Autodesk Inventor part; units mm, degrees
ref_plane "YZ Plane" through (0, 0, 0) normal (1, 0, 0) x (0, 1, 0)
ref_plane "XZ Plane" through (0, 0, 0) normal (0, 1, 0) x (-1, 0, 0)
ref_plane "XY Plane" through (0, 0, 0) normal (0, 0, 1) x (1, 0, 0)
sketch "Sketch1" plane through (0, 0, 0) normal (0, 0, 1) x (1, 0, 0)
  line L0 (0, 0) -> (24, 0)
  line L1 (24, 0) -> (24, -100)
  line L2 (24, -100) -> (0, -100)
  line L3 (0, -100) -> (0, 0)
  dimension "d0" = 24
  dimension "d1" = 100
extrude "Extrusion1" add sketch "Sketch1" along normal blind 2
sketch "Sketch2" plane through (0, 0, 2) normal (0, 0, 1) x (1, 0, 0)
  line L0 (0, -100) -> (24, -100)
  line L1 (0, 0) -> (2, 0)
  line L2 (2, 0) -> (2, -100)
  line L3 (2, -100) -> (0, -100)
  line L4 (0, -100) -> (0, 0)
  line L5 (24, -100) -> (24, 0)
  line L6 (24, 0) -> (22, 0)
  line L7 (22, 0) -> (22, -100)
  line L8 (22, -100) -> (24, -100)
  line L9 (24, -100) -> (24, 0)
  dimension "d4" = 2
  dimension "d5" = 2
extrude "Extrusion2" add sketch "Sketch2" along normal blind 15
sketch "Sketch3" plane through (24, -100, 0) normal (1, 0, 0) x (0, 0, -1)
  circle A0 centre (-8.5, 97) radius 1
  circle A1 centre (-8.5, 69.5) radius 1
  line L0 (-17, 0) -> (-17, 100)
  line L1 (0, 100) -> (-17, 100)
  dimension "d8" = 2
  dimension "d9" = 2
  dimension "d10" = 8.5
  dimension "d11" = 8.5
  dimension "d12" = 27.5
  dimension "d13" = 3
extrude "Extrusion3" cut sketch "Sketch3" against normal up to surface (2 mm away)
sketch "Sketch4" plane through (24, -100, 0) normal (1, 0, 0) x (0, 0, -1)
  line L0 (-17, 100) -> (-17, 0)
  line L1 (-2, 95) -> (-2, 71.5)
  circle A0 centre (-8.5, 97) radius 1
  circle A1 centre (-8.5, 69.5) radius 1
  line L2 (0, 0) -> (0, 100)
  line L3 (-2, 95) -> (-17, 95)
  line L4 (-17, 95) -> (-17, 71.5)
  line L5 (-17, 71.5) -> (-2, 71.5)
  point P0 (-17, 95)
  dimension "d24" = 23.5
  dimension "d104" = 15
  dimension "d105" = 2
  dimension "d106" = 2
extrude "Extrusion4" cut sketch "Sketch4" against normal up to surface (2 mm away) contours L3 L1 L5 L0
sketch "Sketch5" plane through (0, -100, 0) normal (-1, 0, 0) x (0, 0, 1)
  circle A0 centre (8.5, 88.4) radius 2.5
  circle A1 centre (8.5, 97) radius 1
  point P0 (0, 100)
  dimension "d29" = 5
  dimension "d32" = 8.6
  dimension "d33" = 0
extrude "Extrusion5" add sketch "Sketch5" along normal blind 5 contours A0
sketch "Sketch15" plane through (0, 0, 0) normal (0, 1, 0) x (1, 0, 0)
  line L0 (22, -17) -> (24, -17)
  line L1 (0, 0) -> (0, -17)
  line L2 (24, -17) -> (0, -17)
  line L3 (0, -17) -> (0, 0)
  line L4 (0, 0) -> (24, 0)
  line L5 (24, 0) -> (24, -17)
extrude "Extrusion12" add sketch "Sketch15" along normal blind 2
sketch "Sketch16" plane through (24, -100, 17) normal (1, 0, 0) x (0, 0, -1)
  line L0 (0, 100) -> (0, 0)
  line L1 (0, 5) -> (15, 5)
  line L2 (15, 5) -> (15, 28.5)
  line L3 (15, 28.5) -> (0, 28.5)
  line L4 (0, 28.5) -> (0, 5)
  line L5 (17, 0) -> (0, 0)
  circle A0 centre (8.5, 3) radius 1
  circle A1 centre (8.5, 30.5) radius 1
  point P0 (17, 100)
  point P1 (0, 71.5)
  point P2 (7.5, 5)
  point P3 (7.5, 28.5)
  point P4 (0, 28.5)
  dimension "d84" = 15
  dimension "d85" = 23.5
  dimension "d86" = 5
  dimension "d87" = 2
  dimension "d88" = 2
  dimension "d89" = 8.5
  dimension "d90" = 8.5
  dimension "d91" = 2
  dimension "d92" = 2
extrude "Extrusion13" cut sketch "Sketch16" against normal up to surface (2 mm away)
sketch "Sketch17" plane through (0, -100, 0) normal (0, -1, 0) x (1, 0, 0)
  line L0 (24, 4) -> (24, 17)
  line L1 (24, 17) -> (0, 17)
  line L2 (0, 17) -> (0, 0)
  line L3 (0, 0) -> (24, 0)
  line L4 (24, 0) -> (24, 17)
  point P0 (24, 2)
extrude "Extrusion14" add sketch "Sketch17" along normal blind 2
sketch "Sketch18" plane through (0, 2, 0) normal (-1, 0, 0) x (0, 0, 1)
  circle A0 centre (8.5, -90.4) radius 2.5
  line L0 (17, -104) -> (0, -104)
  line L1 (17, -104) -> (17, 0)
  point P0 (0, -2)
  dimension "d97" = 5
  dimension "d98" = 13.6
  dimension "d99" = 8.5
extrude "Extrusion15" add sketch "Sketch18" along normal blind 5
ref_plane "Plano de trabalho3" through (2, -44.5, 2) normal (1, 0, 0) x (0, 0, -1)
sketch "Sketch21" plane through (2, -44.5, 2) normal (1, 0, 0) x (0, 0, -1)
  circle A0 centre (-6.5, -5.5) radius 6
  line L0 (0, 9) -> (-15, 9)
  line L1 (-15, -35.5) -> (-15, 44.5)
  circle A1 centre (-6.4973, 4.5) radius 1.5
  circle A2 centre (-6.5, -15.5) radius 1.5
  line L2 (0, 44.5) -> (-15, 44.5)
  point P0 (2, 44.5)
  point P1 (-15, 0)
  point P2 (-15, 46.5)
  dimension "d122" = 12
  dimension "d124" = 8.5
  dimension "d129" = 3
  dimension "d130" = 3
  dimension "d131" = 10
  dimension "d132" = 10
  dimension "d134" = 50
extrude "Extrusion18" cut sketch "Sketch21" against normal up to surface (2 mm away)
sketch "Esboço22" plane through (0, 0, 2) normal (0, 0, 1) x (1, 0, 0)
  line L0 (22, -71.5) -> (22, -28.5)
  line L1 (22, -38.5) -> (15, -38.5)
  line L2 (15, -38.5) -> (15, -61.5)
  line L3 (15, -61.5) -> (22, -61.5)
  line L4 (22, -61.5) -> (22, -38.5)
  line L5 (24, -28.5) -> (22, -28.5)
  line L6 (22, -71.5) -> (24, -71.5)
  point P0 (0, 0)
  dimension "d142" = 7
  dimension "d143" = 10
  dimension "d144" = 10
extrude "Extrusão19" add sketch "Esboço22" along normal up to surface (15 mm away)
equation "\"d11\" = d10"
equation "\"d90\" = d89"
properties part number "corpo"
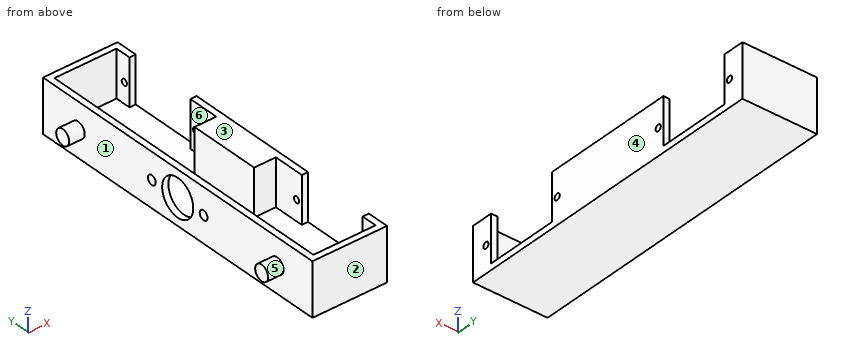
The listing builds one solid part. Answer for the finished solid, in the listing's coordinates (mm). Face numbers are marked on the shaded views. A direction names the side the tool comes from. Coordinates: 2 decimals unless noted, no trailing zeros. Write each loop counter-clockwise with the first axis right and the second up, starting at its lowest first coordinate (ties: lowest second). Pieces come first, ordered by that corner, then holes. Notation, with made-up numbers: M 29.25,8.25 L 55.25,8.25 A37 ccw 55.25,45.25 Z; hole C 0.5,-27.75 d3. An arc over 180 degrees is marked long. Write each question's results on one line, items separated by ' | '.
Item 1: Consider probe 1 along Y at (x, z) = (15.25, 13.5); probe 2 along Y at (x, z) = (10, 13.5); probe 3 along X at (y, z) = (-31, 4.25). Determine where each line is inside the solid, lowest interval first. Write a range as [from, to].
Answer below:
probe 1: [-102, -100], [-61.5, -38.5], [0, 2] | probe 2: [-102, -100], [0, 2] | probe 3: [0, 2], [22, 24]
Item 2: Given P1, Ø1.5, axis at x = 0.5, y = -11, coming from the -Z side; P2, Ø8, axis at y = -23.5, z = 12.5, coming from the +X side; P3, Ø7.5, axis at y = -52.5, z = 6, coming from the -X side, each flat-ended and moving along its own axis, determine where each tip first touches the part or whether it passes through.
Answer below:
P1: z = 0 | P2: x = 2 | P3: x = 0
Item 3: The part is cut by section D-D on y = -50. Determine the outline of the cut face in (x, z), and give its area (3 significant figures).
Answer below:
outline: M 0,0 L 24,0 L 24,17 L 15,17 L 15,2 L 2,2 L 2,2.5 L 0,2.5 Z; M 0,14.5 L 2,14.5 L 2,17 L 0,17 Z | area: 189 mm2
Item 4: Which of the six approach directions +Z, -Z, +X, -X, +Y, -Y give full straight-line access (tool end or side, diameter ignored) to the marked faces 4, 5 and 6?
Answer below:
face 4: +Z, -Z, +X, +Y, -Y | face 5: -X | face 6: +Z
Item 5: The part is cut by section A-A on y = -69.5. Determine the outline of the cut face in (x, z).
Answer below:
outline: M 0,0 L 24,0 L 24,7.5 L 22,7.5 L 22,2 L 2,2 L 2,17 L 0,17 Z; M 22,9.5 L 24,9.5 L 24,17 L 22,17 Z
Item 6: The part is cut by section B-B on x = 18.5. Determine the outline of the cut face in (y, z).
Answer below:
outline: M -102,0 L 2,0 L 2,17 L 0,17 L 0,2 L -38.5,2 L -38.5,17 L -61.5,17 L -61.5,2 L -100,2 L -100,17 L -102,17 Z
Item 7: The part is cut by section C-C on y = -36.5. Determine the outline of the cut face in (x, z).
Answer below:
outline: M 0,0 L 24,0 L 24,17 L 22,17 L 22,2 L 2,2 L 2,17 L 0,17 Z
Item 8: For a pull along Y with two mould halves and no side action, classify the marked faces 1, 2 and 3 as released by +Y, released by -Y, zero draft, split by the parting line, or undercut.
Answer below:
face 1: undercut | face 2: released by -Y | face 3: zero draft
